```python
from build123d import *

# Parameters (mm, degrees)
PAD021_DEPTH  = 30
SKETCH003_R   = 3
HOLE004_DEPTH = 50.001
FILLET008_R   = 14
FILLET009_R   = 3
FILLET010_R   = 2


with BuildPart() as part:
    # Sketch002 → Pad021 (new body)
    with BuildSketch(Plane.YZ):
        Polygon((-25, 50), (-23, 50), (-23, 2), (23, 2), (23, 50), (25, 50), (25, 0), (-25, 0), align=None)
    extrude(amount=PAD021_DEPTH)

    # Sketch003 → Hole004 (cut, through all)
    with BuildSketch(Plane(origin=(0, -25, 0), x_dir=(0, 0, -1), z_dir=(0, -1, 0))):
        with Locations((-35, 15)):
            Circle(SKETCH003_R)
    extrude(amount=-HOLE004_DEPTH, mode=Mode.SUBTRACT)

    # Fillet008
    fillet008_edges = [part.edges().sort_by_distance(p)[0] for p in [
        (30, 24, 50),
        (30, -24, 50),
        (0, -24, 50),
        (0, 24, 50),
    ]]
    fillet(fillet008_edges, radius=FILLET008_R)

    # Fillet009
    fillet009_edges = [part.edges().sort_by_distance(p)[0] for p in [
        (15, -23, 2),
        (15, 23, 2),
    ]]
    fillet(fillet009_edges, radius=FILLET009_R)

    # Fillet010
    fillet010_edges = [part.edges().sort_by_distance(p)[0] for p in [
        (15, 25, 0),
        (15, -25, 0),
    ]]
    fillet(fillet010_edges, radius=FILLET010_R)


solid = part.part
```
Can you work these out from the model? Positions are in its coordinate system, mm. A direction names the side the tool comes from. Coordinates: 2 decimals unless noted, no trailing zeros. Order: outer loops, then holes, each group sorted by start corner. A loop starts at its lowest first (then second) coordinate and runs counter-clockwise, first axis right, second up.
1. Thinking about a two-plate mould opening in Z: for faces 3 (the face through (25.8, -24, 46)), 4 (the face through (13.2, 24, 37.4)), 5 (the face through (15, 23, 27)), which applies, +Z half, -Z half, draft (parallel to the pull), parting line (faces both ways), or undercut?
2. I'm going to push flat-ended pins straight in: pin 1 (9 mm diameter, centred on x = 19, y = -3, fed in from +Z); pin 2 (5.5 mm diameter, centred on x = 15, z = 35, fed in from -Y). Where does each tip first touch, or does it pass through?
3. For faces 1 (the face through (15, 0, 2)), 2 (the face through (15, 25, 26)), which set-ups out of +Z, -Z, +X, -X, +Y, -Y let a thin tool reach every point of the face, with its end or its side?
4. If we section it at D-D (x = 22.75): Please give me the cut outline in (y, z), then the cut area to 3 significant figures.
5. If we section it at C-C (z = 35): Please give me the cut outline in (x, y), then the cut area to 3 significant figures.
6. I need wall thicknesses on line 1 (Y direction, x = 2.75, z = 38); line 2 (X direction, y = -24.2, z = 35); line 3 (Z direction, x = 9.5, y = 5). Which ranges of each line are inside material? Lowest first, please.
7. If we section it at A-A (x = 15): Please give me the cut outline in (y, z), then the cut area to 3 significant figures.
8. If we section it at B-B (z = 16): Please give me the cut outline in (x, y).
Entries:
1. face 3: +Z half
1. face 4: undercut
1. face 5: draft
2. pin 1: stops at z = 2
2. pin 2: passes through
3. face 1: +Z, +X, -X
3. face 2: +Z, -Z, +X, -X, +Y
4. outline: (-25, 2) arc R2 ccw to (-23, 0) - (23, 0) arc R2 ccw to (25, 2) - (25, 48.27) - (23, 48.27) - (23, 5) arc R3 cw to (20, 2) - (-20, 2) arc R3 cw to (-23, 5) - (-23, 48.27) - (-25, 48.27) - close
4. area: 287 mm2
5. outline: (0, -25) - (12, -25) - (12, -23) - (0, -23) - close; (0, 23) - (12, 23) - (12, 25) - (0, 25) - close; (18, -25) - (30, -25) - (30, -23) - (18, -23) - close; (18, 23) - (30, 23) - (30, 25) - (18, 25) - close
5. area: 96.0 mm2
6. line 1: y = -25 to -23, 23 to 25
6. line 2: x = 0 to 12, 18 to 30
6. line 3: z = 0 to 2
7. outline: (-25, 2) arc R2 ccw to (-23, 0) - (23, 0) arc R2 ccw to (25, 2) - (25, 32) - (23, 32) - (23, 5) arc R3 cw to (20, 2) - (-20, 2) arc R3 cw to (-23, 5) - (-23, 32) - (-25, 32) - close; (-25, 38) - (-23, 38) - (-23, 50) - (-25, 50) - close; (23, 38) - (25, 38) - (25, 50) - (23, 50) - close
7. area: 270 mm2
8. outline: (0, -25) - (30, -25) - (30, -23) - (0, -23) - close; (0, 23) - (30, 23) - (30, 25) - (0, 25) - close
